Here's how the part is built. I have some questions about the finished solid (model axes, mm). Coordinates: 2 decimals unless noted, no trailing zeros. Loops run counter-clockwise (first coordinate to the right, second up) from the corner with the lowest first, then second, coordinate; pieces in that order, holes last. Notation, with made-up numbers: (-19.5, 88) - (-4.5, 88) arc R11 ccw to (-4.5, 106) - close; hole circle Ø6 at (9, 27.5). An arc over 180 degrees is marked (long way). Use a Markdown table: item, result.
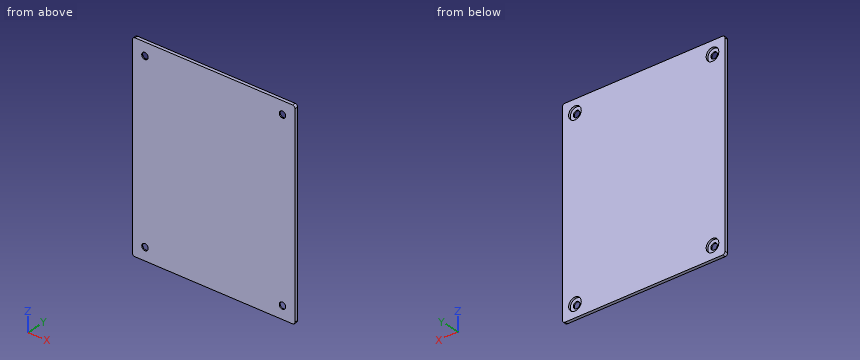
```python
from build123d import *

# Parameters (mm, degrees)
SKETCH1_W                                        = 164.846
SKETCH1_H                                        = 200.152
BOSS_EXTRUDE1_DEPTH                              = 3.175
CBORE_FOR_1_4_SOCKET_HEAD_CAP_SCREW1_D           = 6.5278
CBORE_FOR_1_4_SOCKET_HEAD_CAP_SCREW1_CBORE_D     = 12.827
CBORE_FOR_1_4_SOCKET_HEAD_CAP_SCREW1_CBORE_DEPTH = 2.032
FILLET1_R                                        = 2.54


with BuildPart() as part:
    # Sketch1 → Boss-Extrude1 (new body)
    with BuildSketch(Plane(origin=(0, 0, 0), x_dir=(1, 0, 0), z_dir=(0, 1, 0))):
        Rectangle(SKETCH1_W, SKETCH1_H)
    extrude(amount=BOSS_EXTRUDE1_DEPTH)

    # CBORE for 1/4 Socket Head Cap Screw1 (through all)
    with Locations(Plane(origin=(0, 3.175, 0), x_dir=(-1, 0, 0), z_dir=(0, 1, 0))):
        with Locations((69.723, 87.376), (69.723, -87.376), (-69.723, 87.376), (-69.723, -87.376)):
            CounterBoreHole(CBORE_FOR_1_4_SOCKET_HEAD_CAP_SCREW1_D / 2, CBORE_FOR_1_4_SOCKET_HEAD_CAP_SCREW1_CBORE_D / 2, CBORE_FOR_1_4_SOCKET_HEAD_CAP_SCREW1_CBORE_DEPTH)

    # Fillet1
    fillet1_edges = [part.edges().sort_by_distance(p)[0] for p in [
        (82.423, 1.5875, 100.076),
        (-82.423, 1.5875, 100.076),
        (-82.423, 1.5875, -100.076),
        (82.423, 1.5875, -100.076),
    ]]
    fillet(fillet1_edges, radius=FILLET1_R)


solid = part.part
```
Q1. Will these pins go through, and if not, where does the flat tip stop? P1, Ø8.5, axis at x = -69.723, z = -87.376, coming from the +Y side; P2, Ø5, axis at x = -14.5, z = 30, coming from the -Y side; P3, Ø5, axis at x = 69.723, z = -87.376, coming from the +Y side.
Check values:
| item | result |
|---|---|
| P1 | y = 1.14 |
| P2 | y = 0 |
| P3 | through |
Q2. I want a section at A-A, the plane y = 1.75. Write out the boundary of the cut face in (x, z).
Check values:
| item | result |
|---|---|
| outline | (-82.42, -97.54) arc R2.54 ccw to (-79.88, -100.08) - (79.88, -100.08) arc R2.54 ccw to (82.42, -97.54) - (82.42, 97.54) arc R2.54 ccw to (79.88, 100.08) - (-79.88, 100.08) arc R2.54 ccw to (-82.42, 97.54) - close; hole circle Ø12.83 at (-69.72, -87.38); hole circle Ø12.83 at (-69.72, 87.38); hole circle Ø12.83 at (69.72, -87.38); hole circle Ø12.83 at (69.72, 87.38) |
Q3. Please list where these lines run through material, in increasing order: L1, parallel to X at y = 1.4, z = -90; L2, parallel to X at y = 1.5, z = 88.5. Write a range as from..to.
Check values:
| item | result |
|---|---|
| L1 | -82.42..-75.58, -63.87..63.87, 75.58..82.42 |
| L2 | -82.42..-76.04, -63.41..63.41, 76.04..82.42 |
